from build123d import *

# Parameters (mm, degrees)
SKETCH_1_R      = 28.5
EXTRUDE_1_DEPTH = 30


with BuildPart() as part:
    # 草图1 → 凸台-拉伸1 (new body)
    with BuildSketch(Plane(origin=(0, 0, 0), x_dir=(1, 0, 0), z_dir=(0, 1, 0))):
        with BuildLine():
            Line((28.354893758, -28.5), (100, -28.5))
            Line((100, -28.5), (100, -38.5))
            Line((100, -38.5), (0, -38.5))
            ThreePointArc((0, -38.5), (-38.5, 0), (0, 38.5))
            Line((0, 38.5), (100, 38.5))
            Line((100, 38.5), (100, 28.5))
            Line((100, 28.5), (28.354893758, 28.5))
            ThreePointArc((28.354893758, 28.5), (27.433969621, 27.889741881), (27.637048346, 26.803797468))
            ThreePointArc((27.637048346, 26.803797468), (38.5, 0), (27.637048346, -26.803797468))
            ThreePointArc((27.637048346, -26.803797468), (27.433969621, -27.889741881), (28.354893758, -28.5))
        make_face()
        with Locations(Location((0, 0, 0), (0, 0, 270))):
            Circle(SKETCH_1_R, mode=Mode.SUBTRACT)
    extrude(amount=EXTRUDE_1_DEPTH)


solid = part.part
Here's how the part is built. I have some questions about the finished solid (model axes, mm). A direction names the side the tool comes from. Round coordinates to 2 decimals unless told otherwise and drop trailing zeros. Order: outer loops, then holes, each group sorted by start corner. A loop starts at its lowest first (then second) coordinate and runs counter-clockwise, first axis right, second up. Notation, with made-up numbers: (29.5, 57.25) -> (60.5, 57.25) arc R34 cw to (60.5, 90.25) -> close; hole circle Ø11 at (24.25, -2.5). An arc over 180 degrees is marked (long way). Return JSON: item names as keys, results as strings.
Q1. If we section it at A-A on y = 17.75: List the corners of the cut face in (x, z) for me.
Filled sheet:
{"outline": "(0, -38.5) -> (100, -38.5) -> (100, -28.5) -> (28.35, -28.5) arc R1 cw to (27.64, -26.8) arc R38.5 ccw to (27.64, 26.8) arc R1 cw to (28.35, 28.5) -> (100, 28.5) -> (100, 38.5) -> (0, 38.5) arc R38.5 ccw to start; hole circle Ø57 at (0, 0)"}
Q2. Which directions (+Z, -Z, +X, -X, +Y, -Y) give clear straight access to the entire face, cutting with the end or side of a thin tool? Please do faces 4 (the flat face through (32, 30, -1)), 5 (the flat face through (65, 15, -28.5)).
Filled sheet:
{"face 4": "+Z, -Z, +X, -X, +Y", "face 5": "+X, +Y, -Y"}
Q3. For pin 1 Ø1.5 at (y, z) = (22.5, 26) entering from -X; pin 2 Ø1 at (y, z) = (23, -26) entering from -X; pin 3 Ø1 at (y, z) = (22, 16) entering from -X, each with a flat end and sliding along its axis, tell me the tip position at first contact or that it passes through.
Filled sheet:
{"pin 1": "stops at x = -29.06", "pin 2": "stops at x = -28.84", "pin 3": "stops at x = -35.24"}
Q4. If we mould it in two halves opening along X, with no side actions, what happens to faces 1 (the flat face through (100, 15, 33)), 2 (the flat face through (32, 0, -1)), 3 (the cylindrical face through (-27.82, 14.79, -6.18))? For each: released by +X, released by -X, zero draft, split by the parting line, or undercut.
Filled sheet:
{"face 1": "released by +X", "face 2": "zero draft", "face 3": "undercut"}
Q5. If we section it at D-D on x = 33.5: List the corners of the cut face in (y, z) for me.
Filled sheet:
{"outline": "(0, -38.5) -> (30, -38.5) -> (30, -28.5) -> (0, -28.5) -> close; (0, -18.97) -> (30, -18.97) -> (30, 18.97) -> (0, 18.97) -> close; (0, 28.5) -> (30, 28.5) -> (30, 38.5) -> (0, 38.5) -> close"}
Q6. If we section it at C-C on z = 0: List the corners of the cut face in (x, y) for me.
Filled sheet:
{"outline": "(-38.5, 0) -> (-28.5, 0) -> (-28.5, 30) -> (-38.5, 30) -> close; (28.5, 0) -> (38.5, 0) -> (38.5, 30) -> (28.5, 30) -> close"}
Q7. If we section it at B-B on x = 81.5: List the corners of the cut face in (y, z) for me.
Filled sheet:
{"outline": "(0, -38.5) -> (30, -38.5) -> (30, -28.5) -> (0, -28.5) -> close; (0, 28.5) -> (30, 28.5) -> (30, 38.5) -> (0, 38.5) -> close"}
Q8. I need wall thicknesses on line 1 along Z through (x, y) = (60, 12); line 2 along X through (y, z) = (5.25, -4); line 3 along X through (y, z) = (22.75, 4.5). Which ranges of each line are inside material? Lowest first, please. Write a range as from..to.
Filled sheet:
{"line 1": "z = -38.5..-28.5, 28.5..38.5", "line 2": "x = -38.29..-28.22, 28.22..38.29", "line 3": "x = -38.24..-28.14, 28.14..38.24"}
